CAD build for the part. Positions are in the model's coordinates, mm. Face numbers are marked on the shaded views. A direction names the side the tool comes from. Coordinates: 2 decimals unless noted, no trailing zeros. Loops run counter-clockwise (first coordinate to the right, second up) from the corner with the lowest first, then second, coordinate; pieces in that order, holes last. Notation, with made-up numbers: (12.5, 45.25) - (37.5, 45.25) arc R4 ccw to (37.5, 50.25) - close; hole circle Ø8 at (-2.75, 74). An arc over 180 degrees is marked (long way). Put each result on its own line as item: value.
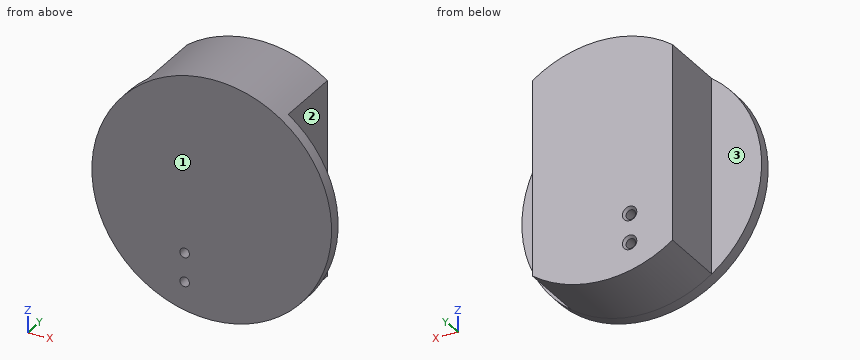
```python
from build123d import *

# Parameters (mm, degrees)
IZIM1_R                     = 50
BASE_DEPTH                  = 5
Y_KSEKLIK_EKSTR_ZYON2_START = 30
Y_KSEKLIK_EKSTR_ZYON2_DEPTH = 30
IZIM2_R                     = 2
BANANA_SLOTU_DEPTH          = 79.89866919
PAH1_SIZE                   = 1


with BuildPart() as part:
    # izim1 → base (new body)
    with BuildSketch(Plane(origin=(0, 0, 0), x_dir=(1, 0, 0), z_dir=(0, 1, 0))):
        with Locations(Location((0, 0, 0), (0, 0, 270))):
            Circle(IZIM1_R)
    extrude(amount=-BASE_DEPTH)

    # izim1_3 → Y_kseklik-Ekstr_zyon2 (add)
    with BuildSketch(Plane(origin=(0, 0, 0), x_dir=(1, 0, 0), z_dir=(0, 1, 0)).offset(Y_KSEKLIK_EKSTR_ZYON2_START)):
        with BuildLine():
            ThreePointArc((29.199046601, 40.588368748), (0, 50), (-29.199046601, 40.588368748))
            Line((-29.199046601, 40.588368748), (-29.199046601, 16.5))
            Line((-29.199046601, 16.5), (-29.199046601, -16.5))
            Line((-29.199046601, -16.5), (-29.199046601, -40.588368748))
            ThreePointArc((-29.199046601, -40.588368748), (0, -50), (29.199046601, -40.588368748))
            Line((29.199046601, -40.588368748), (29.199046601, -16.5))
            Line((29.199046601, -16.5), (29.199046601, 16.5))
            Line((29.199046601, 16.5), (29.199046601, 40.588368748))
        make_face()
    extrude(amount=-Y_KSEKLIK_EKSTR_ZYON2_DEPTH)

    # izim2 → banana slotu (cut, through all)
    with BuildSketch(Plane(origin=(0, 30, 0), x_dir=(1, 0, 0), z_dir=(0, 1, 0))):
        with Locations(Location((-11.3, 36.942764929, 0), (0, 0, 270))):
            Circle(IZIM2_R)
        with Locations(Location((-11.3, 24.942764929, 0), (0, 0, 90))):
            Circle(IZIM2_R)
    extrude(amount=-BANANA_SLOTU_DEPTH, mode=Mode.SUBTRACT)

    # Pah1
    pah1_edges = [part.edges().sort_by_distance(p)[0] for p in [
        (-11.3, 30, -38.942764929),
        (-11.3, 30, -22.942764929),
    ]]
    chamfer(pah1_edges, length=PAH1_SIZE)


solid = part.part
```
Q1. Pin check, flat tips, straight feed: pin 1 Ø8 at (x, y) = (-17, -1) entering from +Z; pin 2 Ø3 at (x, z) = (-11.3, -36.94) entering from +Y; pin 3 Ø10.5 at (x, z) = (43, -4) entering from +Y; pin 4 Ø10 at (y, z) = (9, 17) entering from -X. Stop position of each tip, or through.
Determined:
pin 1: z = 48.28
pin 2: through
pin 3: y = 0
pin 4: x = -29.2
Q2. Slice it at A-A, the plane y = 21. Give the cut face in (x, z).
Determined:
outline: (-29.2, -40.59) arc R50 ccw to (29.2, -40.59) - (29.2, 40.59) arc R50 ccw to (-29.2, 40.59) - close; hole circle Ø4 at (-11.3, -36.94); hole circle Ø4 at (-11.3, -24.94)
Q3. Slice it at D-D, the plane x = 21.5. Give the cut face in (y, z).
Determined:
outline: (-5, -45.14) - (30, -45.14) - (30, 45.14) - (-5, 45.14) - close
Q4. Wall check: L1, parallel to Z at x = -11, y = 10.5 (3 decimals); L2, parallel to X at y = 4, z = -31.5; L3, parallel to Y at x = -30, z = 32. Give the ranges that are in metal, low to high. Write a range as from..to.
Determined:
L1: -48.775..-38.92, -34.965..-26.92, -22.965..48.775
L2: -29.2..29.2
L3: -5..0
Q5. Slice it at C-C, the plane z = 0. Give the cut face in (x, y).
Determined:
outline: (-50, -5) - (50, -5) - (50, 0) - (29.2, 0) - (29.2, 30) - (-29.2, 30) - (-29.2, 0) - (-50, 0) - close
Q6. Tool access for the marked faces 1, 2 and 3: list every direction of +Z, -Z, +X, -X, +Y, -Y with a clear straight run to the whole face (end or side of a thin tool).
Determined:
face 1: +Z, -Z, +X, -X, -Y
face 2: +Z, -Z, +X, +Y
face 3: +Z, -Z, -X, +Y
